from build123d import *

# Parameters (mm, degrees)
BOSS_EXTRUDE1_DEPTH = 30
SKETCH2_R           = 16.5
BOSS_EXTRUDE2_DEPTH = 60
SKETCH3_R           = 15.5
CUT_EXTRUDE1_DEPTH  = 118.763469435


with BuildPart() as part:
    # Sketch1 → Boss-Extrude1 (new body)
    with BuildSketch(Plane(origin=(0, 0, 0), x_dir=(1, 0, 0), z_dir=(0, 1, 0))):
        with BuildLine():
            ThreePointArc((-16.019255805, 10.488088482), (-71.019255805, 0), (-16.019255805, -10.488088482))
            ThreePointArc((-16.019255805, -10.488088482), (38.980744195, 0), (-16.019255805, 10.488088482))
        make_face()
    extrude(amount=BOSS_EXTRUDE1_DEPTH)

    # Sketch2 → Boss-Extrude2 (add)
    with BuildSketch(Plane.XY):
        with Locations(Location((-16.019255805, 15, 0), (0, 0, 245.380016324))):
            Circle(SKETCH2_R)
    extrude(amount=BOSS_EXTRUDE2_DEPTH)

    # Sketch3 → Cut-Extrude1 (cut, through all)
    with BuildSketch(Plane.XY.offset(60)):
        with Locations((-16.019255805, 15)):
            Circle(SKETCH3_R)
    extrude(amount=-CUT_EXTRUDE1_DEPTH, mode=Mode.SUBTRACT)


solid = part.part
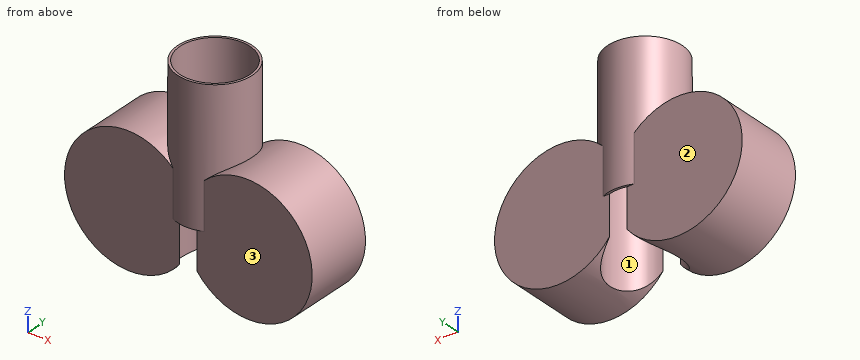
Input: part model. Units: mm. Frame: model coordinates. Face numbers are marked on the shaded views. Coordinates: 2 decimals unless noted, no trailing zeros. Loops run counter-clockwise (first coordinate to the right, second up) from the corner with the lowest first, then second, coordinate; pieces in that order, holes last. Notation, with made-up numbers: (63, -6.5) -> (102, -6.5) arc R14 cw to (102, 0.5) -> close; hole circle Ø8 at (-8.5, 18). An arc over 180 degrees is marked (long way). Write each question's results on one line, items separated by ' | '. Start each with the question number.
Q1. Section A-A, the plane y = 15. Return the cut outline in (x, z), plus the area to 3 significant figures.
Q2. Ray query, line 1 (X direction, y = 15, z = -0.5); line 2 (X direction, y = 15, z = 31); line 3 (X direction, y = 1.5, z = 24.5). Return the intervals inside material, ascending. Write a range as from..to.
Q3. Pull-direction query (Y, two-part tool) for the marked faces 1, 2 and 3; classes: released by +Y, released by -Y, zero draft, split by the parting line, or undercut.
Q4. Section C-C, the plane z = -9. Return the cut outline in (x, y).
Q5. Pin query (flat end, axial travel): pin 1 (3 mm diameter, centred on y = 23, z = 43, fed in from -X) (3 decimals); pin 2 (15.5 mm diameter, centred on x = 1.5, z = -1, fed in from +Y); pin 3 (5 mm diameter, centred on y = 19, z = -14, fed in from +X). Return the tip coordinate at first contact, or that it passes through.
Q6. Section D-D, the plane x = 12. Return the cut outline in (y, z).
Q7. Section B-B, the plane z = 9. Return the cut outline in (x, y).
Found:
1) outline: (-32.52, 26.69) arc R28.5 ccw (long way) to (-31.52, -26.29) -> (-31.52, 60) -> (-32.52, 60) -> close; (-0.52, -26.29) arc R28.5 ccw (long way) to (0.48, 26.69) -> (0.48, 60) -> (-0.52, 60) -> close | area: 3,840 mm2
2) line 1: -71.01..-31.52, -0.52..38.98 | line 2: -32.52..-31.52, -0.52..0.48 | line 3: -57.08..-27.96, -25.51..-23.64, -8.4..-6.53, -4.08..25.04
3) face 1: undercut | face 2: released by +Y | face 3: released by -Y
4) outline: (-69.56, 0) -> (-19.92, 0) arc R15.5 cw to (-19.92, 30) -> (-69.56, 30) -> close; (-12.11, 0) -> (37.52, 0) -> (37.52, 30) -> (-12.11, 30) arc R15.5 cw to start
5) pin 1: x = -31.185 | pin 2: y = 30 | pin 3: x = 36.56
6) outline: (0, -28.46) -> (30, -28.46) -> (30, 28.46) -> (0, 28.46) -> close
7) outline: (-69.56, 0) -> (-22.89, 0) arc R16.5 ccw to (-9.15, 0) -> (37.52, 0) -> (37.52, 30) -> (-9.15, 30) arc R16.5 ccw to (-22.89, 30) -> (-69.56, 30) -> close; hole circle Ø31 at (-16.02, 15)
